Check sheet for the modelled part. Datum: model origin and axes. Units: mm. Round coordinates to 2 decimals unless told otherwise and drop trailing zeros. Write each loop counter-clockwise with the first axis right and the second up, starting at its lowest first coordinate (ties: lowest second). Pieces come first, ordered by that corner, then holes. Notation, with made-up numbers: M 13,-37 L 69,-37 A22 ccw 69,-26 Z; hole C 3,-20 d8. An arc over 180 degrees is marked long. One line per item, written item: value.
from build123d import *

# Parameters (mm, degrees)
F0_W     = 11.938
F0_H     = 17.018
F0_H_2   = 50.8
F0_H_3   = 63.5
F0_W_2   = 25.4
F0_H_4   = 11.938
F1_DEPTH = 11.938


with BuildPart() as f1:
    # F0 (on Front) → F1 (new body)
    with BuildSketch(Plane.XZ):
        with BuildLine():
            Line((0, 152.4), (263.9645430735, 152.4))
            ThreePointArc((263.9645430735, 152.4), (152.4, 263.9645430735), (0, 304.8))
            Line((0, 304.8), (0, 228.6))
            Line((0, 228.6), (0, 152.4))
        make_face()
        with Locations((127.381, 184.6740592089)):
            Rectangle(F0_W, F0_H, mode=Mode.SUBTRACT)
        with Locations((100.457, 203.2)):
            Rectangle(F0_W, F0_H_2, mode=Mode.SUBTRACT)
        with Locations((127.381, 220.091)):
            Rectangle(F0_W, F0_H, mode=Mode.SUBTRACT)
        with BuildLine():
            ThreePointArc((0, 304.8), (-152.4, 263.9645430735), (-263.9645430735, 152.4))
            Line((-263.9645430735, 152.4), (0, 152.4))
            Line((0, 152.4), (0, 228.6))
            Line((0, 228.6), (0, 304.8))
        make_face()
        with Locations((-127.381, 186.309)):
            Rectangle(F0_W, F0_H, mode=Mode.SUBTRACT)
        with Locations((-127.381, 220.091)):
            Rectangle(F0_W, F0_H, mode=Mode.SUBTRACT)
        with Locations((-100.457, 203.2)):
            Rectangle(F0_W, F0_H_2, mode=Mode.SUBTRACT)
        with BuildLine():
            ThreePointArc((-263.9645430735, 152.4), (-78.8880449472, -294.4141918529), (304.8, 0))
            ThreePointArc((304.8, 0), (294.4141918529, 78.8880449472), (263.9645430735, 152.4))
            Line((263.9645430735, 152.4), (0, 152.4))
            Line((0, 152.4), (-263.9645430735, 152.4))
        make_face()
        with Locations((-211.709, -120.65)):
            Rectangle(F0_W, F0_H_3, mode=Mode.SUBTRACT)
        with Locations((-166.878, -119.38)):
            Rectangle(F0_W_2, F0_H_4, mode=Mode.SUBTRACT)
        with Locations((166.878, -119.38)):
            Rectangle(F0_W_2, F0_H_4, mode=Mode.SUBTRACT)
        with Locations((211.709, -120.65)):
            Rectangle(F0_W, F0_H_3, mode=Mode.SUBTRACT)
        with BuildLine():
            ThreePointArc((0, -6.985), (-4.9391408666, 4.9391408666), (6.985, 0))
            ThreePointArc((6.985, 0), (4.9391408666, -4.9391408666), (0, -6.985))
        make_face(mode=Mode.SUBTRACT)
    extrude(amount=F1_DEPTH)


solid = f1.part
Q1. Sectioned sample at C-C on z = -259. Enter the section's corners in (x, y), and give its area (3 significant figures).
Completed:
outline: M -160.69,-11.94 L 160.69,-11.94 L 160.69,0 L -160.69,0 Z
area: 3,840 mm^2
Q2. Sectioned sample at A-A on z = -137. Enter the section's corners in (x, y), and give its area (3 significant figures).
Completed:
outline: M -272.28,-11.94 L -217.68,-11.94 L -217.68,0 L -272.28,0 Z; M -205.74,-11.94 L 205.74,-11.94 L 205.74,0 L -205.74,0 Z; M 217.68,-11.94 L 272.28,-11.94 L 272.28,0 L 217.68,0 Z
area: 6,220 mm^2
Q3. Depth check by flat-ended pin: P1, Ø6, axis at y = -4.5, z = 223.5, coming from the -X side; P2, Ø4, axis at x = -149.5, y = -4, coming from the -Z side; P3, Ø1.5, axis at x = -87, y = -3.5, coming from the -Z side; P4, Ø12, axis at x = -158.5, z = 224.5, coming from the +Y side. Enter the tip coordinate at first touch or a pass-through.
Completed:
P1: x = -210.43
P2: z = -266.73
P3: z = -292.34
P4: y = 0
Q4. Scan lines: line 1 (X direction, y = -9.5, z = 0) (3 decimals); line 2 (Z direction, x = -216.5, y = -11); line 3 (Z direction, x = -211.5, y = -9.25). Record each from-to range of solid material in increasing order. Write a range as [from, to].
Completed:
line 1: [-304.8, -6.985], [6.985, 304.8]
line 2: [-214.55, -152.4], [-88.9, 214.55]
line 3: [-219.48, -152.4], [-88.9, 219.48]
Q5. Sectioned sample at B-B on x = 195. Enter the section's corners in (y, z).
Completed:
outline: M -11.94,-234.26 L 0,-234.26 L 0,234.26 L -11.94,234.26 Z
